The model under review builds one solid part; all positions refer to its coordinate system, in mm. A direction names the side the tool comes from. Give positions to 0.01 mm unless a question says otherwise; leave off trailing zeros. Order: outer loops, then holes, each group sorted by start corner. A loop starts at its lowest first (then second) coordinate and runs counter-clockwise, first axis right, second up.
```python
from build123d import *

# Parameters (mm, degrees)
F0_W     = 100
F0_H     = 50
F1_DEPTH = 20
F2_W     = 45
F2_H     = 50
F3_DEPTH = 50
F4_W     = 25
F4_H     = 60
F5_DEPTH = 50
F6_R     = 10
F7_DEPTH = 45
F8_R     = 7.5
F9_DEPTH = 10
F10_R    = 5
F11_SIZE = 1


with BuildPart() as f1:
    # F0 (on Top) → F1 (new body)
    with BuildSketch(Plane.XY):
        with Locations((50, 25)):
            Rectangle(F0_W, F0_H)
    extrude(amount=F1_DEPTH)

    # F2 (on face) → F3 (join)
    with BuildSketch(Plane.XY.offset(20)):
        with Locations((22.5, 25)):
            Rectangle(F2_W, F2_H)
    extrude(amount=F3_DEPTH)

    # F4 (on face) → F5 (cut, through all)
    with BuildSketch(Plane.XZ):
        with Locations((22.5, 30)):
            Rectangle(F4_W, F4_H)
    extrude(amount=-F5_DEPTH, mode=Mode.SUBTRACT)

    # F6 (on face) → F7 (cut, through all)
    with BuildSketch(Plane(origin=(0, 0, 0), x_dir=(0, -1, 0), z_dir=(-1, 0, 0))):
        with Locations((-25, 40)):
            Circle(F6_R)
    extrude(amount=-F7_DEPTH, mode=Mode.SUBTRACT)

    # F8 (on face) → F9 (cut, through all)
    with BuildSketch(Plane.XY.offset(70)):
        with Locations((22.5, 25)):
            Circle(F8_R)
    extrude(amount=-F9_DEPTH, mode=Mode.SUBTRACT)

    # F10
    f10_edges = [f1.edges().sort_by_distance(p)[0] for p in [
        (0, 25, 70),
        (0, 50, 35),
        (22.5, 50, 70),
    ]]
    fillet(f10_edges, radius=F10_R)

    # F11
    f11_edges = [f1.edges().sort_by_distance(p)[0] for p in [
        (0, 0, 32.5),
        (25, 0, 70),
        (45, 0, 45),
        (35, 0, 30),
        (22.5, 0, 60),
        (10, 0, 30),
    ]]
    chamfer(f11_edges, length=F11_SIZE)


solid = f1.part
```
Item 1: Take a section at B-B (x = 22.5). Give the boundary of the cut face in (y, z), and give its area (3 significant figures).
Values found:
outline: (0, 61) - (1, 60) - (17.5, 60) - (17.5, 70) - (1, 70) - (0, 69) - close; (32.5, 60) - (50, 60) - (50, 65) arc R5 ccw to (45, 70) - (32.5, 70) - close
area: 344 mm2
Item 2: Draft analysis for pull direction X (two halves, no side actions). For faces 1 (the flat face through (29, 18, 70)), 2 (the flat face through (10, 25.2, 29.6)), 3 (the flat face through (0, 18, 32)), 4 (the flat face through (35, 25.2, 29.6)), state which applies: released by +X, released by -X, zero draft, split by the parting line, or undercut.
Values found:
face 1: zero draft
face 2: undercut
face 3: released by -X
face 4: undercut
Item 3: Take a section at A-A (z = 5). Give the boundary of the cut face in (x, y).
Values found:
outline: (0, 1) - (1, 0) - (9, 0) - (10, 1) - (10, 50) - (5, 50) arc R5 ccw to (0, 45) - close; (35, 1) - (36, 0) - (100, 0) - (100, 50) - (35, 50) - close
Item 4: Take a section at C-C (y = 31). Give the boundary of the cut face in (x, z).
Values found:
outline: (0, 0) - (10, 0) - (10, 32) - (0, 32) - close; (0, 48) - (10, 48) - (10, 60) - (18, 60) - (18, 70) - (5, 70) arc R5 ccw to (0, 65) - close; (27, 60) - (35, 60) - (35, 48) - (45, 48) - (45, 70) - (27, 70) - close; (35, 0) - (100, 0) - (100, 20) - (45, 20) - (45, 32) - (35, 32) - close
Item 5: For line 1 (X direction, y = 3.5, z = 3); line 2 (Y direction, x = 22.5, z = 65); line 3 (Z direction, x = 6.5, y = 25), list the stretches that pass through material, from the lowest coordinate up.
Values found:
line 1: x = 0 to 10, 35 to 100
line 2: y = 0 to 17.5, 32.5 to 50
line 3: z = 0 to 30, 50 to 70
Item 6: Take a section at D-D (z = 46). Give the boundary of the cut face in (x, y), and give its area (3 significant figures).
Values found:
outline: (0, 1) - (1, 0) - (9, 0) - (10, 1) - (10, 17) - (0, 17) - close; (0, 33) - (10, 33) - (10, 50) - (5, 50) arc R5 ccw to (0, 45) - close; (35, 1) - (36, 0) - (44, 0) - (45, 1) - (45, 17) - (35, 17) - close; (35, 33) - (45, 33) - (45, 50) - (35, 50) - close
area: 673 mm2
Item 7: Clearance check with a flat-ended pin moving along its axis: pin 1 Ø14.5 at (y, z) = (34, 46.5) entering from +X. State where the tip first meets the part, or that it passes through.
Values found:
pin 1: stops at x = 45
Item 8: For faces 5 (the flat face through (100, 25, 10)), 6 (the flat face through (16.8, 19.7, 60)), 7 (the flat face through (45, 25.2, 50.2)), list the 3-axis set-ups (+Z, -Z, +X, -X, +Y, -Y) from which the entire face can be reached by the end or side of a thin tool; tool diameter is ignored.
Values found:
face 5: +Z, -Z, +X, +Y, -Y
face 6: -Z, +Y, -Y
face 7: +Z, +X, +Y, -Y
